Geometry: final body of the model. Coordinates: model frame, mm. Face numbers are marked on the shaded views. A direction names the side the tool comes from. Give positions to 0.01 mm unless a question says otherwise; leave off trailing zeros. Order: outer loops, then holes, each group sorted by start corner. A loop starts at its lowest first (then second) coordinate and runs counter-clockwise, first axis right, second up. Notation, with made-up numbers: (-5.75, 0) -> (3.25, 0) arc R27 ccw to (3.25, 22) -> close; hole circle Ø8 at (74, 63.5). An arc over 180 degrees is marked (long way). Write item = value, one per line.
```python
from build123d import *

# Parameters (mm, degrees)
BASPROSKE_W             = 4
BASPROSKE_H             = 18
TOOTHCUT_DEPTH          = 26.768197453
TEETHCUTS_COUNT         = 16
TEETHCUTS_ANGLE         = 337.5
BORSKE_R                = 3
BORE_DEPTH              = 50.0000508
SALIENTE_EXTRUIR2_DEPTH = 4
MATRIZC1_COUNT          = 25
CROQUIS5_R              = 4
CROQUIS5_R_2            = 1.5
SALIENTE_EXTRUIR3_DEPTH = 2
CROQUIS6_R              = 2.85
CORTAR_EXTRUIR4_DEPTH   = 0.8


with BuildPart() as part:
    # BasProSke → Base-Revolve (revolve)
    with BuildSketch(Plane(origin=(0, 0, 0), x_dir=(1, 0, 0), z_dir=(0, 1, 0)), mode=Mode.PRIVATE) as base_revolve_sk:
        with Locations((2, 9)):
            Rectangle(BASPROSKE_W, BASPROSKE_H)
    revolve(base_revolve_sk.sketch.rotate(Axis((-10, 0, 0), (1, 0, 0)), 180), axis=Axis((-10, 0, 0), (1, 0, 0)))

    # TooCutSke → ToothCut (cut, through all)
    with BuildSketch(Plane(origin=(0, 0, 0), x_dir=(0, 0, -1), z_dir=(1, 0, 0))):
        with BuildLine():
            ThreePointArc((1.03434411, 13.459313997), (0, 13.499), (-1.03434411, 13.459313997))
            ThreePointArc((-1.03434411, 13.459313997), (-1.635143665, 15.806872195), (-3.065655864, 17.762792553))
            ThreePointArc((-3.065655864, 17.762792553), (0, 18.0254), (3.065655864, 17.762792553))
            ThreePointArc((3.065655864, 17.762792553), (1.635143665, 15.806872195), (1.03434411, 13.459313997))
        make_face()
    toothcut = extrude(amount=TOOTHCUT_DEPTH, mode=Mode.SUBTRACT)

    # TeethCuts: ToothCut ×16 about axis
    teethcuts_axis = Axis((-10, 0, 0), (1, 0, 0))
    for i in range(1, TEETHCUTS_COUNT):
        add(toothcut.rotate(teethcuts_axis, i * TEETHCUTS_ANGLE / (TEETHCUTS_COUNT - 1)), mode=Mode.SUBTRACT)

    # BorSke → Bore (cut, symmetric)
    with BuildSketch(Plane(origin=(0, 0, 0), x_dir=(0, 0, -1), z_dir=(1, 0, 0))):
        with Locations(Location((0, 0, 0), (0, 0, 180))):
            Circle(BORSKE_R)
    extrude(amount=BORE_DEPTH, both=True, mode=Mode.SUBTRACT)

    # Croquis4 → Saliente-Extruir2 (add, through all)
    with BuildSketch(Plane.ZY):
        with BuildLine():
            Line((-0.266547398, 2.686810839), (-0.504049329, 2.957352579))
            ThreePointArc((-0.504049329, 2.957352579), (-0.296163775, 2.985345377), (-0.08683031, 2.998743153))
            Line((-0.08683031, 2.998743153), (-0.266547398, 2.686810839))
        make_face()
    saliente_extruir2 = extrude(amount=-SALIENTE_EXTRUIR2_DEPTH)

    # MatrizC1: Saliente-Extruir2 ×25 about axis
    matrizc1_axis = Axis((0, 0, 0), (1, 0, 0))
    for i in range(1, MATRIZC1_COUNT):
        add(saliente_extruir2.rotate(matrizc1_axis, i * 360 / MATRIZC1_COUNT))

    # Croquis5 → Saliente-Extruir3 (add)
    with BuildSketch(Plane.ZY):
        with Locations(Location((0, 0, 0), (0, 0, 180))):
            Circle(CROQUIS5_R)
        Circle(CROQUIS5_R_2, mode=Mode.SUBTRACT)
    extrude(amount=SALIENTE_EXTRUIR3_DEPTH)

    # Croquis6 → Cortar-Extruir4 (cut)
    with BuildSketch(Plane.ZY.offset(2)):
        Circle(CROQUIS6_R)
    extrude(amount=-CORTAR_EXTRUIR4_DEPTH, mode=Mode.SUBTRACT)


solid = part.part
```
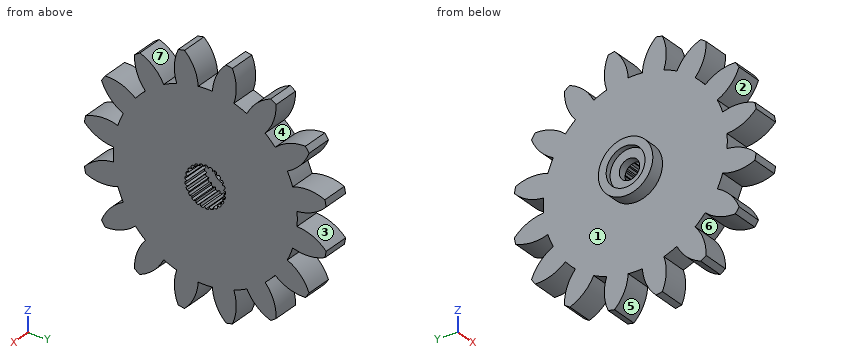
1) Reachability of the marked faces 1, 2, 3 and 4 from +Z, -Z, +X, -X, +Y, -Y: full face, straight path, thin tool, end or side. Return the list, or none.
Check sheet entries:
face_1 = -X
face_2 = +X, -X, -Y
face_3 = +X, -X, +Y
face_4 = +X, -X
2) Mould query, pull axis Z, two halves, no side actions, for the marked faces 5, 6 and 7. Classes: +Z half, -Z half, draft (parallel to the pull), parting line (faces both ways), or undercut.
Check sheet entries:
face_5 = -Z half
face_6 = undercut
face_7 = +Z half
3) Section query B-B (x = -0.75). Output: boundary loops of the cut face in (y, z), plus the area to 3 significant figures.
Check sheet entries:
outline = circle Ø8 at (0, 0); hole circle Ø3 at (0, 0)
area = 43.2 mm²
4) Section query A-A (z = -14). Output: boundary loops of the cut face in (x, y).
Check sheet entries:
outline = (0, -10.38) -> (4, -10.38) -> (4, -7.58) -> (0, -7.58) -> close; (0, -4.48) -> (4, -4.48) -> (4, -1.09) -> (0, -1.09) -> close; (0, 1.09) -> (4, 1.09) -> (4, 4.48) -> (0, 4.48) -> close; (0, 7.58) -> (4, 7.58) -> (4, 10.38) -> (0, 10.38) -> close
5) Section query D-D (z = -7.5). Output: boundary loops of the cut face in (x, y), plus the area to 3 significant figures.
Check sheet entries:
outline = (0, -13.92) -> (4, -13.92) -> (4, 13.92) -> (0, 13.92) -> close
area = 111 mm²
6) Line query: line 1 (Y direction, x = -0.45, z = 0); line 2 (Y direction, x = 1.35, z = 13); line 3 (Y direction, x = -1.4, z = 0). Output: solid intervals per line, ascending. Write a range as from..to.
Check sheet entries:
line_1 = -4..-1.5, 1.5..4
line_2 = -10.22..-6.68, -4.25..4.25, 6.68..10.22
line_3 = -4..-2.85, 2.85..4
7) First-contact query: P1, Ø4, axis at y = 0, z = 0, coming from the -X side; P2, Ø2, axis at x = -0.5, z = -8, coming from the -Y side; P3, Ø3, axis at y = 9, z = -3, coming from the -X side; P4, Ø6.5, axis at y = 0.5, z = -0.5, coming from the +X side. Flat tips, straight axial feed; report the tip coordinate or a pass-through.
Check sheet entries:
P1 = -1.2
P2 = -14.89
P3 = 0
P4 = 4
8) Section query C-C (z = 11.5). Output: boundary loops of the cut face in (x, y).
Check sheet entries:
outline = (0, -9.65) -> (4, -9.65) -> (4, 9.65) -> (0, 9.65) -> close
